The listing builds one solid part. Answer for the finished solid, in the listing's coordinates (mm). A direction names the side the tool comes from. Round coordinates to 2 decimals unless told otherwise and drop trailing zeros. Order: outer loops, then holes, each group sorted by start corner. A loop starts at its lowest first (then second) coordinate and runs counter-clockwise, first axis right, second up. Notation, with made-up numbers: (61, -4.5) -> (67, -4.5) arc R15 ccw to (67, 12.5) -> close; hole circle Ø7 at (-30.75, -26.75). An arc over 180 degrees is marked (long way). Answer in a Markdown table with one row per item. Add a question column.
```python
from build123d import *

# Parameters (mm, degrees)
SKETCH1_R           = 12.09
SKETCH1_R_2         = 1.75
BOSS_EXTRUDE1_DEPTH = 10
SKETCH2_R           = 2.4
SKETCH2_R_2         = 1.3
CUT_EXTRUDE1_DEPTH  = 40.007683858


with BuildPart() as part:
    # Sketch1 → Boss-Extrude1 (new body)
    # profile 1 of 17: a face of its own
    with BuildSketch(Plane.XY):
        Circle(SKETCH1_R)
        Circle(SKETCH1_R_2, mode=Mode.SUBTRACT)
    # profile 2 of 17: a face of its own
    with BuildSketch(Plane.XY):
        with BuildLine():
            Line((30.75, 4), (14.142164609, 3.746702505))
            Line((14.142164609, 3.746702505), (14.211728743, 3.487085624))
            ThreePointArc((14.211728743, 3.487085624), (13.144626757, 2.65424773), (11.903927815, 2.112960617))
            ThreePointArc((11.903927815, 2.112960617), (11.986568374, 1.578061664), (12.04518576, 1.04))
            ThreePointArc((12.04518576, 1.04), (13.383704325, 0.838273314), (14.63, 0.31))
            Line((14.63, 0.31), (14.63, -0.31))
            ThreePointArc((14.63, -0.31), (13.383704325, -0.838273314), (12.04518576, -1.04))
            ThreePointArc((12.04518576, -1.04), (11.986568374, -1.578061664), (11.903927815, -2.112960617))
            ThreePointArc((11.903927815, -2.112960617), (13.144626757, -2.65424773), (14.211728743, -3.487085624))
            Line((14.211728743, -3.487085624), (14.142164609, -3.746702505))
            Line((14.142164609, -3.746702505), (30.75, -4))
            ThreePointArc((30.75, -4), (34.75, 0), (30.75, 4))
        make_face()
        with Locations((30.75, 0)):
            Circle(SKETCH1_R_2, mode=Mode.SUBTRACT)
    # profile 3 of 17: a face of its own
    with BuildSketch(Plane.XY):
        with BuildLine():
            ThreePointArc((-11.365584201, -4.122086336), (-11.67804324, -3.129122255), (-11.903927815, -2.112960617))
            ThreePointArc((-11.903927815, -2.112960617), (-13.144626757, -2.65424773), (-14.211728743, -3.487085624))
            Line((-14.211728743, -3.487085624), (-14.051260935, -4.085959636))
            ThreePointArc((-14.051260935, -4.085959636), (-12.71070456, -4.273667417), (-11.365584201, -4.122086336))
        make_face()
    # profile 4 of 17: a face of its own
    with BuildSketch(Plane.XY):
        with BuildLine():
            ThreePointArc((-12.04518576, -1.04), (-12.09, 0), (-12.04518576, 1.04))
            ThreePointArc((-12.04518576, 1.04), (-13.383704325, 0.838273314), (-14.63, 0.31))
            Line((-14.63, 0.31), (-14.63, -0.31))
            ThreePointArc((-14.63, -0.31), (-13.383704325, -0.838273314), (-12.04518576, -1.04))
        make_face()
    # profile 5 of 17: a face of its own
    with BuildSketch(Plane.XY):
        with BuildLine():
            ThreePointArc((-11.903927815, 2.112960617), (-11.67804324, 3.129122255), (-11.365584201, 4.122086336))
            ThreePointArc((-11.365584201, 4.122086336), (-12.71070456, 4.273667417), (-14.051260935, 4.085959636))
            Line((-14.051260935, 4.085959636), (-14.211728743, 3.487085624))
            ThreePointArc((-14.211728743, 3.487085624), (-13.144626757, 2.65424773), (-11.903927815, 2.112960617))
        make_face()
    # profile 6 of 17: a face of its own
    with BuildSketch(Plane.XY):
        with BuildLine():
            ThreePointArc((-10.951436862, 5.12192646), (-10.470247132, 6.045), (-9.911436862, 6.9232593))
            ThreePointArc((-9.911436862, 6.9232593), (-11.171491285, 7.417818147), (-12.514951657, 7.583467875))
            Line((-12.514951657, 7.583467875), (-12.824951657, 7.046532125))
            ThreePointArc((-12.824951657, 7.046532125), (-12.009764599, 5.965886177), (-10.951436862, 5.12192646))
        make_face()
    # profile 7 of 17: a face of its own
    with BuildSketch(Plane.XY):
        with BuildLine():
            ThreePointArc((-9.252623584, 7.781841479), (-8.548920985, 8.548920985), (-7.781841479, 9.252623584))
            ThreePointArc((-7.781841479, 9.252623584), (-8.870959341, 10.05645683), (-10.125769107, 10.564175311))
            Line((-10.125769107, 10.564175311), (-10.564175311, 10.125769107))
            ThreePointArc((-10.564175311, 10.125769107), (-10.05645683, 8.870959341), (-9.252623584, 7.781841479))
        make_face()
    # profile 8 of 17: a face of its own
    with BuildSketch(Plane.XY):
        with BuildLine():
            ThreePointArc((-6.9232593, 9.911436862), (-6.045, 10.470247132), (-5.12192646, 10.951436862))
            ThreePointArc((-5.12192646, 10.951436862), (-5.965886177, 12.009764599), (-7.046532125, 12.824951657))
            Line((-7.046532125, 12.824951657), (-7.583467875, 12.514951657))
            ThreePointArc((-7.583467875, 12.514951657), (-7.417818147, 11.171491285), (-6.9232593, 9.911436862))
        make_face()
    # profile 9 of 17: a face of its own
    with BuildSketch(Plane.XY):
        with BuildLine():
            ThreePointArc((-4.122086336, 11.365584201), (-3.129122255, 11.67804324), (-2.112960617, 11.903927815))
            ThreePointArc((-2.112960617, 11.903927815), (-2.65424773, 13.144626757), (-3.487085624, 14.211728743))
            Line((-3.487085624, 14.211728743), (-4.085959636, 14.051260935))
            ThreePointArc((-4.085959636, 14.051260935), (-4.273667417, 12.71070456), (-4.122086336, 11.365584201))
        make_face()
    # profile 10 of 17: a face of its own
    with BuildSketch(Plane.XY):
        with BuildLine():
            Line((0.31, 14.63), (-0.31, 14.63))
            ThreePointArc((-0.31, 14.63), (-0.838273314, 13.383704325), (-1.04, 12.04518576))
            ThreePointArc((-1.04, 12.04518576), (0, 12.09), (1.04, 12.04518576))
            ThreePointArc((1.04, 12.04518576), (0.838273314, 13.383704325), (0.31, 14.63))
        make_face()
    # profile 11 of 17: a face of its own
    with BuildSketch(Plane.XY):
        with BuildLine():
            ThreePointArc((3.487085624, 14.211728743), (2.65424773, 13.144626757), (2.112960617, 11.903927815))
            ThreePointArc((2.112960617, 11.903927815), (3.129122255, 11.67804324), (4.122086336, 11.365584201))
            ThreePointArc((4.122086336, 11.365584201), (4.273667417, 12.71070456), (4.085959636, 14.051260935))
            Line((4.085959636, 14.051260935), (3.487085624, 14.211728743))
        make_face()
    # profile 12 of 17: a face of its own
    with BuildSketch(Plane.XY):
        with BuildLine():
            ThreePointArc((7.046532125, 12.824951657), (5.965886177, 12.009764599), (5.12192646, 10.951436862))
            ThreePointArc((5.12192646, 10.951436862), (6.045, 10.470247132), (6.9232593, 9.911436862))
            ThreePointArc((6.9232593, 9.911436862), (7.417818147, 11.171491285), (7.583467875, 12.514951657))
            Line((7.583467875, 12.514951657), (7.046532125, 12.824951657))
        make_face()
    # profile 13 of 17: a face of its own
    with BuildSketch(Plane.XY):
        with BuildLine():
            ThreePointArc((10.125769107, 10.564175311), (8.870959341, 10.05645683), (7.781841479, 9.252623584))
            ThreePointArc((7.781841479, 9.252623584), (8.548920985, 8.548920985), (9.252623584, 7.781841479))
            ThreePointArc((9.252623584, 7.781841479), (10.05645683, 8.870959341), (10.564175311, 10.125769107))
            Line((10.564175311, 10.125769107), (10.125769107, 10.564175311))
        make_face()
    # profile 14 of 17: a face of its own
    with BuildSketch(Plane.XY):
        with BuildLine():
            ThreePointArc((12.514951657, 7.583467875), (11.171491285, 7.417818147), (9.911436862, 6.9232593))
            ThreePointArc((9.911436862, 6.9232593), (10.470247132, 6.045), (10.951436862, 5.12192646))
            ThreePointArc((10.951436862, 5.12192646), (12.009764599, 5.965886177), (12.824951657, 7.046532125))
            Line((12.824951657, 7.046532125), (12.514951657, 7.583467875))
        make_face()
    # profile 15 of 17: a face of its own
    with BuildSketch(Plane.XY):
        with BuildLine():
            Line((14.142164609, 3.746702505), (11.507813792, 3.706524213))
            ThreePointArc((11.507813792, 3.706524213), (11.732956682, 2.916475184), (11.903927815, 2.112960617))
            ThreePointArc((11.903927815, 2.112960617), (13.144626757, 2.65424773), (14.211728743, 3.487085624))
            Line((14.211728743, 3.487085624), (14.142164609, 3.746702505))
        make_face()
    # profile 16 of 17: a face of its own
    with BuildSketch(Plane.XY):
        with BuildLine():
            ThreePointArc((14.63, 0.31), (13.383704325, 0.838273314), (12.04518576, 1.04))
            ThreePointArc((12.04518576, 1.04), (12.078791244, 0.520482544), (12.09, 0))
            ThreePointArc((12.09, 0), (12.078791244, -0.520482544), (12.04518576, -1.04))
            ThreePointArc((12.04518576, -1.04), (13.383704325, -0.838273314), (14.63, -0.31))
            Line((14.63, -0.31), (14.63, 0.31))
        make_face()
    # profile 17 of 17: a face of its own
    with BuildSketch(Plane.XY):
        with BuildLine():
            Line((11.507813792, -3.706524213), (14.142164609, -3.746702505))
            Line((14.142164609, -3.746702505), (14.211728743, -3.487085624))
            ThreePointArc((14.211728743, -3.487085624), (13.144626757, -2.65424773), (11.903927815, -2.112960617))
            ThreePointArc((11.903927815, -2.112960617), (11.732956682, -2.916475184), (11.507813792, -3.706524213))
        make_face()
    extrude(amount=BOSS_EXTRUDE1_DEPTH)

    # Sketch2 → Cut-Extrude1 (cut, through all)
    with BuildSketch(Plane.XY.offset(10)):
        Circle(SKETCH2_R)
        with Locations((4.5, 0)):
            Circle(SKETCH2_R_2)
        with Locations((-4.5, 0)):
            Circle(SKETCH2_R_2)
    extrude(amount=-CUT_EXTRUDE1_DEPTH, mode=Mode.SUBTRACT)


solid = part.part
```
1. For faces 4 (the cylindrical face through (-11.988, -1.571, 4.93)), 5 (the cylindrical face through (-7.35, 9.6, 4.93)), 6 (the cylindrical face through (1.586, 11.986, 4.93)), determine the directions among +Z, -Z, +X, -X, +Y, -Y from which every point of the face is accessible in a straight line to the end or side of a thin tool.
2. The part is cut by section A-A (z = 7.25). Give the number of separate pieces and of enclosed holes in the cut face, then the cut area to 3 significant figures.
3. The part is cut by section B-B (y = -6). Give the vertices of the cut face in (x, z).
4. The mould has two halves that part along X. Classify faces 1 (the cylindrical face through (4.63, 11.17, 4.93)), 2 (the cylindrical face through (-10.066, 8.888, 4.93)), 3 (the cylindrical face through (11.996, 5.952, 4.93)): released by +X, released by -X, zero draft, split by the parting line, or undercut.
5. Each of these flat-tipped pins is pushed along its axis until it touches: pin 1 (3 mm diameter, centred on y = -6.5, z = 7, fed in from +X); pin 2 (3 mm diameter, centred on x = 28, z = 1, fed in from -Y); pin 3 (3 mm diameter, centred on x = 28.5, z = 7.5, fed in from +Y). Where does it stop, or does it pass through?
6. Straight lines are drawn through the part: line 1 along Y through (x, z) = (0, 5.5); line 2 along X through (y, z) = (0.5, 1.5); line 3 along Y through (x, z) = (12.5, 4.25). For each, find the intervals that lie inside material, in ascending order.
Report:
| question | item | result |
|---|---|---|
| 1 | face 4 | +Z, -Z, -X |
| 1 | face 5 | +Z, -Z |
| 1 | face 6 | +Z, -Z, +Y |
| 2 | separate pieces | 1 |
| 2 | enclosed holes | 4 |
| 2 | area | 640 mm^2 |
| 3 | outline | (-10.5, 0) -> (10.5, 0) -> (10.5, 10) -> (-10.5, 10) -> close |
| 4 | face 1 | undercut |
| 4 | face 2 | released by -X |
| 4 | face 3 | released by +X |
| 5 | pin 1 | stops at x = 11.01 |
| 5 | pin 2 | stops at y = -3.98 |
| 5 | pin 3 | stops at y = 3.99 |
| 6 | line 1 | y = -12.09 to -2.4, 2.4 to 14.63 |
| 6 | line 2 | x = -14.27 to -5.7, -3.3 to -2.35, 2.35 to 3.3, 5.7 to 29.07, 32.43 to 34.72 |
| 6 | line 3 | y = -3.72 to 3.72, 6.55 to 7.58 |
